Geometry: final body of the model. Coordinates: model frame, mm. Face numbers are marked on the shaded views. A direction names the side the tool comes from. Coordinates: 2 decimals unless noted, no trailing zeros. Loops run counter-clockwise (first coordinate to the right, second up) from the corner with the lowest first, then second, coordinate; pieces in that order, holes last. Notation, with made-up numbers: (12, 63) - (37, 63) arc R18 ccw to (37, 71) - close; hole circle Ø2 at (48, 50). An arc over 180 degrees is marked (long way). Return JSON: item names as keys, results as strings.
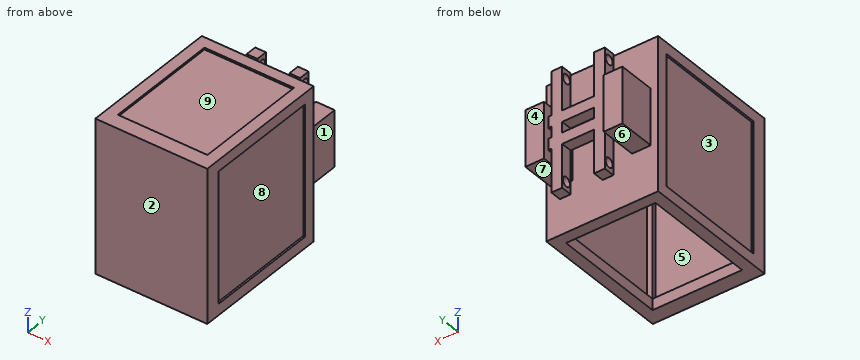
from build123d import *

# Parameters (mm, degrees)
SKETCH2_W            = 480
SKETCH2_H            = 700
BOSS_EXTRUDE1_DEPTH  = 60
SKETCH3_W            = 600
SKETCH3_H            = 820
SKETCH3_W_2          = 480
SKETCH3_H_2          = 700
BOSS_EXTRUDE4_DEPTH  = 80
SKETCH5_W            = 60
SKETCH5_H            = 60
BOSS_EXTRUDE5_DEPTH  = 610
SKETCH7_W            = 600
SKETCH7_H            = 820
BOSS_EXTRUDE6_DEPTH  = 60
BOSS_EXTRUDE7_DEPTH  = 670
SKETCH21_W           = 100
SKETCH21_H           = 300
BOSS_EXTRUDE13_DEPTH = 200
SKETCH28_W           = 60
SKETCH28_H           = 60
BOSS_EXTRUDE18_DEPTH = 520
SKETCH29_W           = 57.5339273
SKETCH29_H           = 60
BOSS_EXTRUDE19_DEPTH = 320
SKETCH30_R           = 25
CUT_EXTRUDE1_DEPTH   = 320


with BuildPart() as part:
    # Sketch2 → Boss-Extrude1 (new body)
    with BuildSketch(Plane(origin=(0, 0, 0), x_dir=(1, 0, 0), z_dir=(0, 1, 0))):
        Rectangle(SKETCH2_W, SKETCH2_H)
    extrude(amount=BOSS_EXTRUDE1_DEPTH)

    # Sketch3 → Boss-Extrude4 (add)
    with BuildSketch(Plane(origin=(0, 0, 0), x_dir=(1, 0, 0), z_dir=(0, 1, 0))):
        Rectangle(SKETCH3_W, SKETCH3_H)
        Rectangle(SKETCH3_W_2, SKETCH3_H_2, mode=Mode.SUBTRACT)
    extrude(amount=BOSS_EXTRUDE4_DEPTH)

    # Sketch5 → Boss-Extrude5 (add)
    with BuildSketch(Plane(origin=(0, 80, 0), x_dir=(1, 0, 0), z_dir=(0, 1, 0))):
        with Locations((270, 380)):
            Rectangle(SKETCH5_W, SKETCH5_H)
        with Locations((-270, 380)):
            Rectangle(SKETCH5_W, SKETCH5_H)
        with Locations((270, -380)):
            Rectangle(SKETCH5_W, SKETCH5_H)
        with Locations((-270, -380)):
            Rectangle(SKETCH5_W, SKETCH5_H)
    extrude(amount=BOSS_EXTRUDE5_DEPTH)

    # Sketch7 → Boss-Extrude6 (add)
    with BuildSketch(Plane(origin=(0, 690, 0), x_dir=(1, 0, 0), z_dir=(0, 1, 0))):
        Rectangle(SKETCH7_W, SKETCH7_H)
    extrude(amount=BOSS_EXTRUDE6_DEPTH)

    # Sketch10 → Boss-Extrude7 (add)
    with BuildSketch(Plane(origin=(0, 80, 0), x_dir=(1, 0, 0), z_dir=(0, 1, 0))):
        Polygon((270, -380), (-270, -380), (-270, 380), (-290, 380), (-290, -400), (290, -400), (290, 380), (270, 380), align=None)
    extrude(amount=BOSS_EXTRUDE7_DEPTH)

    # Sketch21 → Boss-Extrude13 (add)
    with BuildSketch(Plane(origin=(0, 750, 0), x_dir=(1, 0, 0), z_dir=(0, 1, 0))):
        with Locations((-210, 0)):
            Rectangle(SKETCH21_W, SKETCH21_H)
        with Locations((210, 0)):
            Rectangle(SKETCH21_W, SKETCH21_H)
    extrude(amount=BOSS_EXTRUDE13_DEPTH)

    # Sketch28 → Boss-Extrude18 (add)
    with BuildSketch(Plane(origin=(260, 0, 0), x_dir=(0, 0, -1), z_dir=(1, 0, 0))):
        with Locations((58.262274835, 890)):
            Rectangle(SKETCH28_W, SKETCH28_H)
        with Locations((-58.262274835, 890)):
            Rectangle(SKETCH28_W, SKETCH28_H)
    extrude(amount=-BOSS_EXTRUDE18_DEPTH)

    # Sketch29 → Boss-Extrude19 (add, symmetric)
    with BuildSketch(Plane.XY):
        with Locations((-114.414059972, 890)):
            Rectangle(SKETCH29_W, SKETCH29_H)
        with Locations((114.414059972, 890)):
            Rectangle(SKETCH29_W, SKETCH29_H)
    extrude(amount=BOSS_EXTRUDE19_DEPTH, both=True)

    # Sketch30 → Cut-Extrude1 (cut, symmetric)
    with BuildSketch(Plane(origin=(0, 0, 0), x_dir=(0, 0, -1), z_dir=(1, 0, 0))):
        with Locations((-271.32477079, 890)):
            Circle(SKETCH30_R)
        with Locations((271.32477079, 890)):
            Circle(SKETCH30_R)
    extrude(amount=CUT_EXTRUDE1_DEPTH, both=True, mode=Mode.SUBTRACT)


solid = part.part
Item 1: Section query C-C, the plane y = 890. Count the separate pieces of the cut face and the enclosed holes in it, and give its area (3 significant figures).
Worked out:
{"separate pieces": "5", "enclosed holes": "3", "area": "147,000 mm^2"}
Item 2: Mould query, pull axis Y, two halves, no side actions, for the marked faces 1, 2, 3 and 4. Classes: +Y half, -Y half, draft (parallel to the pull), parting line (faces both ways), or undercut.
Worked out:
{"face 1": "draft", "face 2": "-Y half", "face 3": "undercut", "face 4": "+Y half"}
Item 3: Ray query, probe 1 along Y at (x, z) = (-146.5, -209); probe 2 along Y at (x, z) = (242, -311); probe 3 along X at (y, z) = (276, 353.5). Return the intervals inside material, ascending. Write a range as from..to.
Worked out:
{"probe 1": "0..60, 690..750", "probe 2": "0..80, 690..750", "probe 3": "-300..-240, 240..300"}
Item 4: Section query D-D, the plane x = -19. Return loops of the section in (y, z), and give its area (3 significant figures).
Worked out:
{"outline": "(0, -410) - (80, -410) - (80, -350) - (60, -350) - (60, 350) - (80, 350) - (80, 380) - (690, 380) - (690, -410) - (750, -410) - (750, 410) - (690, 410) - (690, 400) - (80, 400) - (80, 410) - (0, 410) - close; (860, -88.26) - (920, -88.26) - (920, -28.26) - (860, -28.26) - close; (860, 28.26) - (920, 28.26) - (920, 88.26) - (860, 88.26) - close", "area": "120,000 mm^2"}
Item 5: Section query B-B, the plane z = -184.5. Return loops of the section in (x, y).
Worked out:
{"outline": "(-300, 0) - (300, 0) - (300, 80) - (290, 80) - (290, 690) - (300, 690) - (300, 750) - (-300, 750) - (-300, 690) - (-290, 690) - (-290, 80) - (-300, 80) - close; (-143.18, 860) - (-85.65, 860) - (-85.65, 920) - (-143.18, 920) - close; (85.65, 860) - (143.18, 860) - (143.18, 920) - (85.65, 920) - close; hole (-270, 80) - (-240, 80) - (-240, 60) - (240, 60) - (240, 80) - (270, 80) - (270, 690) - (-270, 690) - close"}
Item 6: Reachability of the marked faces 5, 6, 7, 8 and 9 from +Z, -Z, +X, -X, +Y, -Y: full face, straight path, thin tool, end or side. Return the list, or none.
Worked out:
{"face 5": "none", "face 6": "-Z, -X, +Y", "face 7": "-Z, +X, +Y", "face 8": "+X", "face 9": "+Z"}
Item 7: First-contact query: pin 1 Ø10 at (x, z) = (-215.5, 182.5) entering from +Y; pin 2 Ø18.5 at (x, y) = (-149, 878) entering from -Z; pin 3 Ø5 at (x, y) = (-114.5, 532) entering from +Z. Flat tips, straight axial feed; report the tip coordinate or a pass-through.
Worked out:
{"pin 1": "y = 750", "pin 2": "z = -320", "pin 3": "z = 400"}
Item 8: Section query A-A, the plane x = -116.5. Return loops of the section in (y, z), and give its area (3 significant figures).
Worked out:
{"outline": "(0, -410) - (80, -410) - (80, -350) - (60, -350) - (60, 350) - (80, 350) - (80, 380) - (690, 380) - (690, -410) - (750, -410) - (750, 410) - (690, 410) - (690, 400) - (80, 400) - (80, 410) - (0, 410) - close; (860, -320) - (920, -320) - (920, 320) - (860, 320) - close; hole circle Ø50 at (890, -271.32); hole circle Ø50 at (890, 271.32)", "area": "147,000 mm^2"}
